from build123d import *

# Parameters (mm, degrees)
SKETCH_2_W          = 48
SKETCH_2_H          = 110
EXTRUDE_1_DEPTH     = 3
SKETCH_3_W          = 4
SKETCH_3_H          = 110
EXTRUDE_2_DEPTH     = 20
SKETCH_4_R          = 1.6
CUT_EXTRUDE_1_DEPTH = 77.537572473
SKETCH_5_W          = 25
SKETCH_5_H          = 23
CUT_EXTRUDE_2_DEPTH = 77.537572473


with BuildPart() as part:
    # 草图2 → 凸台-拉伸1 (new body)
    with BuildSketch(Plane(origin=(0, 0, 0), x_dir=(1, 0, 0), z_dir=(0, 1, 0))):
        Rectangle(SKETCH_2_W, SKETCH_2_H)
    extrude(amount=EXTRUDE_1_DEPTH)

    # 草图3 → 凸台-拉伸2 (add)
    with BuildSketch(Plane(origin=(0, 3, 0), x_dir=(1, 0, 0), z_dir=(0, 1, 0))):
        with Locations((-22, 0)):
            Rectangle(SKETCH_3_W, SKETCH_3_H)
        with Locations((22, 0)):
            Rectangle(SKETCH_3_W, SKETCH_3_H)
    extrude(amount=EXTRUDE_2_DEPTH)

    # 草图4 → 切除-拉伸1 (cut, through all)
    with BuildSketch(Plane.ZY.offset(24)):
        with Locations((0, 14)):
            Circle(SKETCH_4_R)
        with Locations((-25, 14)):
            Circle(SKETCH_4_R)
        with Locations(Location((25, 14, 0), (0, 0, 180))):
            Circle(SKETCH_4_R)
    extrude(amount=-CUT_EXTRUDE_1_DEPTH, mode=Mode.SUBTRACT)

    # 草图5 → 切除-拉伸2 (cut, through all)
    with BuildSketch(Plane(origin=(24, 0, 0), x_dir=(0, 0, -1), z_dir=(1, 0, 0))):
        with Locations((-42.5, 11.5)):
            Rectangle(SKETCH_5_W, SKETCH_5_H)
    extrude(amount=-CUT_EXTRUDE_2_DEPTH, mode=Mode.SUBTRACT)


solid = part.part
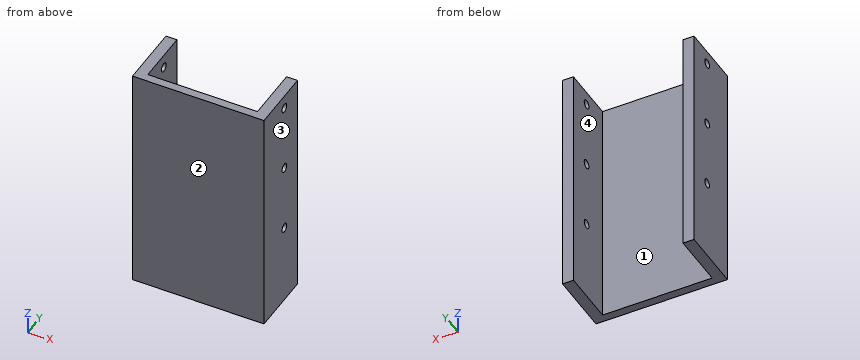
Design review of the part built by this model. Coordinates are the model's own, in mm. Face numbers are marked on the shaded views. Coordinates: 2 decimals unless noted, no trailing zeros. Write each loop counter-clockwise with the first axis right and the second up, starting at its lowest first coordinate (ties: lowest second). Pieces come first, ordered by that corner, then holes. Notation, with made-up numbers: (61.25, 12.5) -> (65.25, 12.5) arc R19 ccw to (65.25, 33.5) -> close; hole circle Ø10 at (57, 30.25). An arc over 180 degrees is marked (long way). Write each question's results on one line, items separated by ' | '. Start each with the question number.
(1) For line 1 along X through (y, z) = (16, -38.5); line 2 along Y through (x, z) = (21.15, 25); line 3 along Y through (x, z) = (-15, -24), list the stretches that pass through material, from the lowest coordinate up. Write a range as from..to.
(2) Take a section at B-B on y = 6.25. Write out the cut boundary in (x, z).
(3) Clearance check with flat-ended pins moving along their axes: P1, Ø5, axis at y = 14, z = 25, coming from the +X side; P2, Ø12, axis at x = 8.5, z = -4.5, coming from the +Y side. State where each tip first meets the part, or that it passes through.
(4) Take a section at C-C on z = 10. Write out the cut boundary in (x, y), and give its area (3 significant figures).
(5) Take a section at A-A on z = 0. Write out the cut boundary in (x, y), and give its area (3 significant figures).
(6) Take a section at D-D on y = 14. Give the number of separate pieces and of enclosed holes in the cut face, and give its area (3 significant figures).
(7) The part is to be moulded in two halves that separate along X. For the marked faces 1, 2, 3 and 4, say which applies: pulls with the +X half, pulls with the -X half, needs draft (parallel to the pull), parting line crosses it, or undercut.
Results found:
1) line 1: x = -24..-20, 20..24 | line 2: y = 0..12.4, 15.6..23 | line 3: y = 0..3
2) outline: (-24, -55) -> (-20, -55) -> (-20, 30) -> (-24, 30) -> close; (20, -55) -> (24, -55) -> (24, 30) -> (20, 30) -> close
3) P1: stops at x = 24 | P2: stops at y = 3
4) outline: (-24, 0) -> (24, 0) -> (24, 23) -> (20, 23) -> (20, 3) -> (-20, 3) -> (-20, 23) -> (-24, 23) -> close | area: 304 mm2
5) outline: (-24, 0) -> (24, 0) -> (24, 12.4) -> (20, 12.4) -> (20, 3) -> (-20, 3) -> (-20, 12.4) -> (-24, 12.4) -> close; (-24, 15.6) -> (-20, 15.6) -> (-20, 23) -> (-24, 23) -> close; (20, 15.6) -> (24, 15.6) -> (24, 23) -> (20, 23) -> close | area: 278 mm2
6) separate pieces: 8 | enclosed holes: 0 | area: 603 mm2
7) face 1: undercut | face 2: needs draft | face 3: pulls with the +X half | face 4: undercut
